Answer from the drawing. Dimensions are ordinates in mm from the lowest x, y and z of the part. A direction names the side the tool comes from. Give positions to 0.01 mm unless a question says otherwise; leave off trailing zeros. Loops run counter-clockwise (first coordinate to the right, second up) from the corner with the lowest first, then second, coordinate; pieces in that order, holes last.
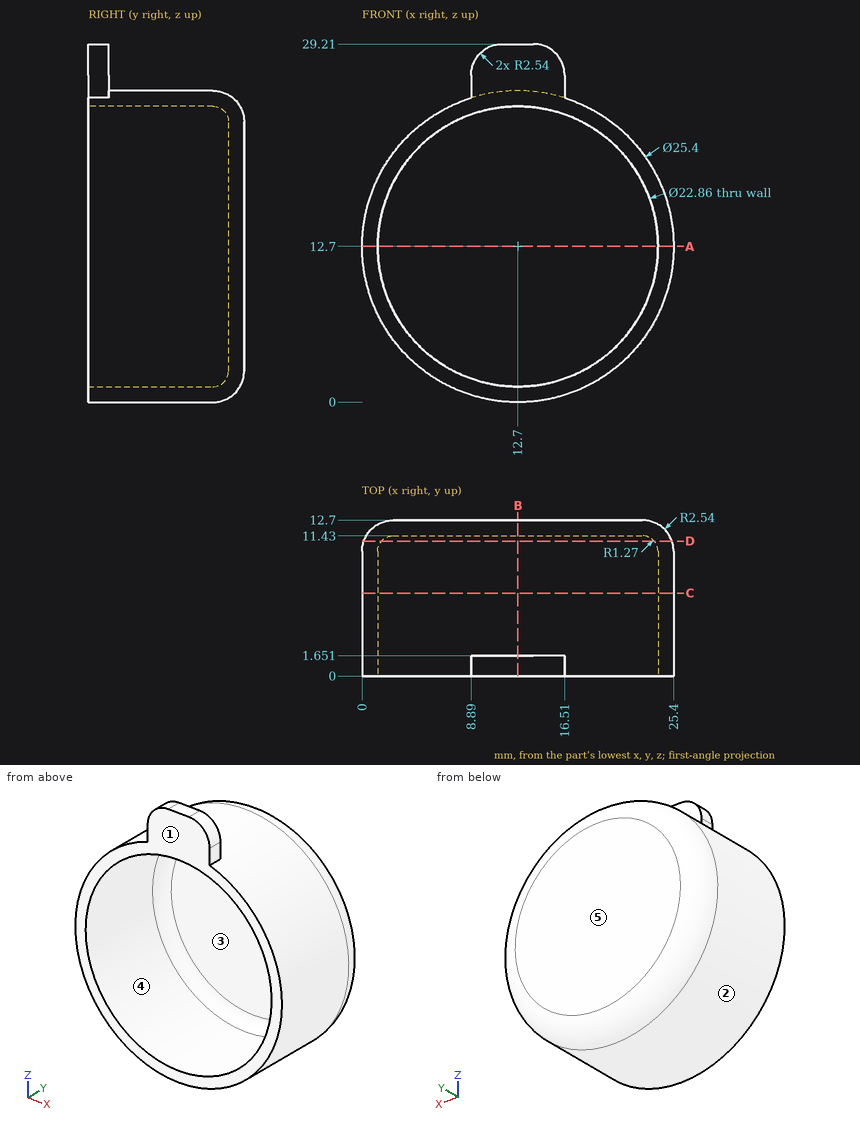
Item 1: Flat-ended cylindrical pins translate along their axes: pin 1 Ø1 at (x, y) = (15, 5) entering from +Z; pin 2 Ø5 at (x, y) = (20, 2) entering from +Z; pin 3 Ø3 at (x, y) = (22, 6) entering from +Z; pin 4 Ø1.5 at (x, z) = (2.5, 10) entering from +Y. Find the tip coordinate at first contact, or state that the pin passes through.
Item 2: Find section C-C, the plane y = 6.75. Write down the section's boundary in (x, z), plus the area to 3 significant figures.
Item 3: For the marked faces 4 and 5, determine the directions among +Z, -Z, +X, -X, +Y, -Y from which every point of the face is accessible in a straight line to the end or side of a thin tool.
Item 4: Determine the mould class of the marked faces 1, 2 and 3 for opening direction Z: released by +Z, released by -Z, zero draft, split by the parting line, or undercut.
Item 5: Consider line 1 (X direction, y = 7, z = 12.7); line 2 (Y direction, x = 15, z = 20.25); line 3 (Z direction, x = 14, y = 1.5). Determine where each line is inside the solid, lowest interval first.
Item 6: Find section D-D, the plane y = 11. Write down the section's boundary in (x, z).
Item 7: Find section B-B, the plane x = 12.7. Write down the section's boundary in (y, z), plus the area to 3 significant figures.
Item 8: Find section A-A, the plane z = 12.7. Write down the section's boundary in (x, y), plus the area to 3 significant figures.
Ans:
1. pin 1: stops at z = 25.27
1. pin 2: stops at z = 24.46
1. pin 3: stops at z = 22.72
1. pin 4: stops at y = 12.7
2. outline: circle Ø25.4 at (12.7, 12.7); hole circle Ø22.86 at (12.7, 12.7)
2. area: 96.3 mm2
3. face 4: -Y
3. face 5: +Z, -Z, +X, -X, +Y
4. face 1: zero draft
4. face 2: split by the parting line
4. face 3: undercut
5. line 1: x = 0 to 1.27, 24.13 to 25.4
5. line 2: y = 11.43 to 12.7
5. line 3: z = 0.07 to 1.34, 24.06 to 29.21
6. outline: circle Ø25.11 at (12.7, 12.7); hole circle Ø22.23 at (12.7, 12.7)
7. outline: (0, 0) - (10.16, 0) arc R2.54 ccw to (12.7, 2.54) - (12.7, 22.86) arc R2.54 ccw to (10.16, 25.4) - (1.65, 25.4) - (1.65, 29.21) - (0, 29.21) - (0, 24.13) - (10.16, 24.13) arc R1.27 cw to (11.43, 22.86) - (11.43, 2.54) arc R1.27 cw to (10.16, 1.27) - (0, 1.27) - close
7. area: 65.5 mm2
8. outline: (0, 0) - (1.27, 0) - (1.27, 10.16) arc R1.27 cw to (2.54, 11.43) - (22.86, 11.43) arc R1.27 cw to (24.13, 10.16) - (24.13, 0) - (25.4, 0) - (25.4, 10.16) arc R2.54 ccw to (22.86, 12.7) - (2.54, 12.7) arc R2.54 ccw to (0, 10.16) - close
8. area: 59.2 mm2
